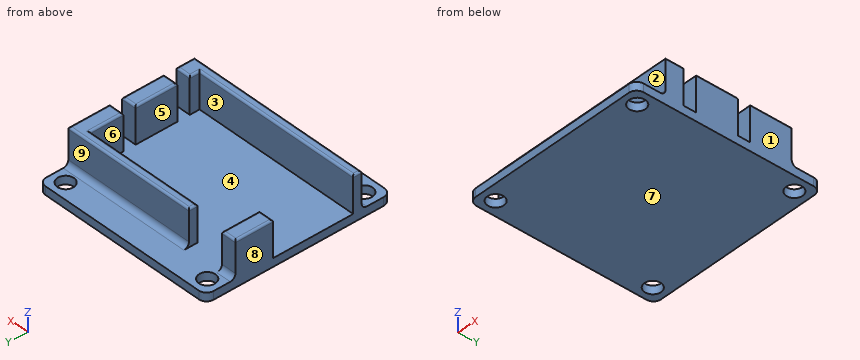
```python
from build123d import *

# Parameters (mm, degrees)
F0_R     = 1.6
F1_DEPTH = 1.6
F2_W     = 2.9
F2_H     = 8.1
F2_H_2   = 1.65
F3_DEPTH = 7
F4_R     = 1
F5_R     = 0.4


with BuildPart() as f1:
    # F0 (on Top) → F1 (new body)
    with BuildSketch(Plane.XY):
        with BuildLine():
            ThreePointArc((-18, -16.5), (-17.5606601718, -17.5606601718), (-16.5, -18))
            Line((-16.5, -18), (16.5, -18))
            ThreePointArc((16.5, -18), (17.5606601718, -17.5606601718), (18, -16.5))
            Line((18, -16.5), (18, 16.5))
            ThreePointArc((18, 16.5), (17.5606601718, 17.5606601718), (16.5, 18))
            Line((16.5, 18), (-16.5, 18))
            ThreePointArc((-16.5, 18), (-17.5606601718, 17.5606601718), (-18, 16.5))
            Line((-18, 16.5), (-18, -16.5))
        make_face()
        with Locations((-15.25, -15.25)):
            Circle(F0_R, mode=Mode.SUBTRACT)
        with Locations((15.25, -15.25)):
            Circle(F0_R, mode=Mode.SUBTRACT)
        with Locations((-15.25, 15.25)):
            Circle(F0_R, mode=Mode.SUBTRACT)
        with Locations((15.25, 15.25)):
            Circle(F0_R, mode=Mode.SUBTRACT)
    extrude(amount=F1_DEPTH)

    # F2 (on face) → F3 (join)
    with BuildSketch(Plane.XY.offset(1.6)):
        Polygon((15.1, -10.6), (-15.1, -10.6), (-15.1, -12.25), (18, -12.25), (18, -8.7), (15.1, -8.7), align=None)
        with Locations((16.55, -2.25)):
            Rectangle(F2_W, F2_H)
        Polygon((-8, 12.25), (-8, 10.6), (15.1, 10.6), (15.1, 4.2), (18, 4.2), (18, 12.25), align=None)
        Polygon((-18, 4.95), (-15.1, 4.95), (-15.1, 10.6), (-15.1, 12.25), (-18, 12.25), align=None)
        with Locations((-16.55, -11.425)):
            Rectangle(F2_W, F2_H_2)
    extrude(amount=F3_DEPTH)

    # F4
    f4_edges = [f1.edges().sort_by_distance(p)[0] for p in [
        (0, -12.25, 1.6),
        (5, 12.25, 1.6),
        (-16.55, 12.25, 1.6),
    ]]
    fillet(f4_edges, radius=F4_R)

    # F5
    f5_edges = [f1.edges().sort_by_distance(p)[0] for p in [
        (5, 12.25, 8.6),
        (3.55, 10.6, 8.6),
        (-15.1, 8.6, 8.6),
        (-18, 8.6, 8.6),
        (-16.55, 12.25, 8.6),
        (-8, 11.425, 8.6),
        (-16.55, 4.95, 8.6),
        (-1.45, -10.6, 8.6),
        (0, -12.25, 8.6),
        (16.55, -8.7, 8.6),
        (18, -10.475, 8.6),
        (15.1, -9.65, 8.6),
        (16.55, -6.3, 8.6),
        (15.1, -2.25, 8.6),
        (18, -2.25, 8.6),
        (16.55, 1.8, 8.6),
        (16.55, 4.2, 8.6),
        (15.1, 7.4, 8.6),
        (18, 8.225, 8.6),
        (-18, -11.425, 8.6),
    ]]
    fillet(f5_edges, radius=F5_R)


solid = f1.part
```
Check sheet for the modelled part. Datum: model origin and axes. Units: mm. Face numbers are marked on the shaded views. A direction names the side the tool comes from. Coordinates: 2 decimals unless noted, no trailing zeros. Order: outer loops, then holes, each group sorted by start corner. A loop starts at its lowest first (then second) coordinate and runs counter-clockwise, first axis right, second up. Notation, with made-up numbers: (64.5, 73) -> (68.5, 73) arc R20 ccw to (68.5, 90) -> close; hole circle Ø11 at (-35.75, 25.5). An arc over 180 degrees is marked (long way). Write item = value, one per line. Start each with the question number.
1) Cross-section at B-B (y = -15.25). Enter the section's corners in (x, z), then the cut area to 3 significant figures.
2) Cross-section at A-A (z = 6). Enter the section's corners in (x, y), then the cut area to 3 significant figures.
3) Material ranges on L1, parallel to Y at x = 15.25, z = 1.15; L2, parallel to Y at x = 6.5, z = 5; L3, parallel to Y at x = 16.5, z = 2.75, recorded low to high.
4) Access from +Z, -Z, +X, -X, +Y, -Y to the whole of each face (thin tool, end or side, straight path). Record for the marked faces 5, 6, 7, 8 and 9.
5) Cross-section at C-C (x = -10.5). Enter the section's corners in (y, z), then the cut area to 3 significant figures.
6) Mould release check, pull along Y, two halves, no side actions. Record for the marked faces 1, 2, 3 and 4: +Y half, -Y half, draft (parallel to the pull), parting line (faces both ways), or undercut.
7) Cross-section at D-D (x = 9). Enter the section's corners in (y, z).
8) Go/stop test with flat-tipped pins: P1, Ø1, axis at y = -9, z = 3.5, coming from the -X side; P2, Ø2, axis at x = 0.5, z = 6, coming from the -Y side; P3, Ø2.5, axis at x = 1, y = -15.5, coming from the +Z side; P4, Ø2.5, axis at x = 15.25, y = -15.25, coming from the +Z side. Record where each tip stops, or that it passes through.
Ans:
q1.outline = (-18, 0) -> (-16.85, 0) -> (-16.85, 1.6) -> (-18, 1.6) -> close; (-13.65, 0) -> (13.65, 0) -> (13.65, 1.6) -> (-13.65, 1.6) -> close; (16.85, 0) -> (18, 0) -> (18, 1.6) -> (16.85, 1.6) -> close
q1.area = 47.4 mm²
q2.outline = (-18, -12.25) -> (18, -12.25) -> (18, -8.7) -> (15.1, -8.7) -> (15.1, -10.6) -> (-18, -10.6) -> close; (-18, 4.95) -> (-15.1, 4.95) -> (-15.1, 12.25) -> (-18, 12.25) -> close; (-8, 10.6) -> (15.1, 10.6) -> (15.1, 4.2) -> (18, 4.2) -> (18, 12.25) -> (-8, 12.25) -> close; (15.1, -6.3) -> (18, -6.3) -> (18, 1.8) -> (15.1, 1.8) -> close
q2.area = 171 mm²
q3.L1 = -18 to -16.85, -13.65 to 13.65, 16.85 to 18
q3.L2 = -12.25 to -10.6, 10.6 to 12.25
q3.L3 = -12.25 to -8.7, -6.3 to 1.8, 4.2 to 12.25
q4.face_5 = +Z, -X
q4.face_6 = +Z
q4.face_7 = -Z, +X, -X, +Y, -Y
q4.face_8 = +Z, -Z, -X, +Y, -Y
q4.face_9 = +Z, +X, -X, +Y
q5.outline = (-18, 0) -> (18, 0) -> (18, 1.6) -> (-10.6, 1.6) -> (-10.6, 8.2) arc R0.4 ccw to (-11, 8.6) -> (-11.85, 8.6) arc R0.4 ccw to (-12.25, 8.2) -> (-12.25, 2.6) arc R1 cw to (-13.25, 1.6) -> (-18, 1.6) -> close
q5.area = 69.3 mm²
q6.face_1 = draft
q6.face_2 = -Y half
q6.face_3 = undercut
q6.face_4 = undercut
q7.outline = (-18, 0) -> (18, 0) -> (18, 1.6) -> (13.25, 1.6) arc R1 cw to (12.25, 2.6) -> (12.25, 8.2) arc R0.4 ccw to (11.85, 8.6) -> (11, 8.6) arc R0.4 ccw to (10.6, 8.2) -> (10.6, 1.6) -> (-10.6, 1.6) -> (-10.6, 8.2) arc R0.4 ccw to (-11, 8.6) -> (-11.85, 8.6) arc R0.4 ccw to (-12.25, 8.2) -> (-12.25, 2.6) arc R1 cw to (-13.25, 1.6) -> (-18, 1.6) -> close
q8.P1 = 15.1
q8.P2 = -12.25
q8.P3 = 1.6
q8.P4 = through
